Build history of the part. All positions in model axes, mm. A direction names the side the tool comes from. Give positions to 0.01 mm unless a question says otherwise; leave off trailing zeros. Order: outer loops, then holes, each group sorted by start corner. A loop starts at its lowest first (then second) coordinate and runs counter-clockwise, first axis right, second up. Notation, with made-up numbers: (-23, 32.25) -> (-10, 32.25) arc R10 ccw to (-10, 43.25) -> close; hole circle Ø4 at (23, 85). An arc over 180 degrees is marked (long way). One line per item, written item: value. Start each with the question number.
(1) Pin check, flat tips, straight feed: pin 1 (4 mm diameter, centred on x = -12, z = -3, fed in from +Y); pin 2 (2 mm diameter, centred on x = -15.5, z = 0.5, fed in from -Y); pin 3 (2 mm diameter, centred on y = -11, z = 0, fed in from -X). Stop position of each tip, or through.
(2) Saw through at C-C on z = -3. Give the cut face in (x, y).
(3) Saw through at D-D on z = 3. Give the cut face in (x, y).
(4) Two-plate mould, pull along X, no slides. Class faces 1 (the flat face through (6.2, 0.4, 0)), 2 (the cylindrical face through (-0.325, -0.084, 1.536)), 3 (the cylindrical face through (-29.97, 1.32, -1.97)): +X half, -X half, draft (parallel to the pull), parting line (faces both ways), or undercut.
(5) Probe line 1 (Z direction, x = 0, y = 1.25); line 2 (Z direction, x = 4, y = 18.5); line 3 (X direction, y = 2.5, z = 3). List the from-to ranges inside material, lowest first.
(6) Saw through at B-B on y = 0. Give the cut face in (x, z).
(7) Which spindle directions (+Z, -Z, +X, -X, +Y, -Y) get a long thin tool onto all of the face, cutting with end or side? Do faces 4 (the flat face through (0, 0, 6)), 5 (the cylindrical face through (5.54, -2.3, 2.96)). Say none if no direction does.
(8) Saw through at A-A on x = 0. Give the cut face in (y, z).
```python
from build123d import *

# Parameters (mm, degrees)
F0_R     = 30
F0_R_2   = 6
F1_DEPTH = 4
F2_DEPTH = 6
F3_R     = 1.5
F4_DEPTH = 12.5


with BuildPart() as f1:
    # F0 (on Top) → F1 (new body)
    with BuildSketch(Plane.XY):
        Circle(F0_R)
        Circle(F0_R_2, mode=Mode.SUBTRACT)
        Circle(F0_R_2)
    extrude(amount=-F1_DEPTH)

    # F0 (on Top) → F2 (join)
    with BuildSketch(Plane.XY):
        Circle(F0_R_2)
    extrude(amount=F2_DEPTH)

    # F3 (on Front) → F4 (cut, symmetric)
    with BuildSketch(Plane.XZ):
        with Locations((0, 3)):
            Circle(F3_R)
    extrude(amount=F4_DEPTH, both=True, mode=Mode.SUBTRACT)


solid = f1.part
```
Results below:
1. pin 1: stops at y = 28.28
1. pin 2: stops at y = -26.19
1. pin 3: stops at x = -28.28
2. outline: circle Ø60 at (0, 0)
3. outline: (-1.5, -5.81) -> (-1.5, 5.81) arc R6 ccw to start; (1.5, -5.81) arc R6 ccw to (1.5, 5.81) -> close
4. face 1: draft
4. face 2: undercut
4. face 3: parting line
5. line 1: z = -4 to 1.5, 4.5 to 6
5. line 2: z = -4 to 0
5. line 3: x = -5.45 to -1.5, 1.5 to 5.45
6. outline: (-30, -4) -> (30, -4) -> (30, 0) -> (6, 0) -> (6, 6) -> (-6, 6) -> (-6, 0) -> (-30, 0) -> close; hole circle Ø3 at (0, 3)
7. face 4: +Z, +X, -X, +Y, -Y
7. face 5: +Z
8. outline: (-30, -4) -> (30, -4) -> (30, 0) -> (6, 0) -> (6, 1.5) -> (-6, 1.5) -> (-6, 0) -> (-30, 0) -> close; (-6, 4.5) -> (6, 4.5) -> (6, 6) -> (-6, 6) -> close
